Part model, mm, in its own coordinate system. A direction names the side the tool comes from. Give positions to 0.01 mm unless a question says otherwise; leave off trailing zeros. Write each loop counter-clockwise with the first axis right and the second up, starting at its lowest first coordinate (ties: lowest second). Pieces come first, ordered by that corner, then holes. Notation, with made-up numbers: M 72,81.25 L 91,81.25 A20 cw 91,117.25 Z; hole C 26,3.25 d8. An arc over 180 degrees is marked long. Answer as CSV lines item,"result". Start each with the question number.
Item 1: Wall check: L1, parallel to X at y = -10.25, z = 8.5; L2, parallel to Y at x = 2.25, z = 7.75; L3, parallel to X at y = 5.75, z = 7. Give the ranges that are in metal, low to high. Write a range as from..to.
Item 2: Pin check, flat tips, straight feed: pin 1 (4.5 mm diameter, centred on x = 10, y = -6.5, fed in from +Z); pin 2 (2 mm diameter, centred on y = 11.5, z = 7, fed in from -X); pin 3 (2 mm diameter, centred on x = -14.5, z = 6.5, fed in from +Y). Stop position of each tip, or through.
Item 3: 3-axis set-ups, long thin cutter, end or side, ignore diameter. For faces 1 (the flat face through (-13, -1, 6)), 2 (the flat face through (8.4, -5, 7.016)), 3 (the flat face through (-14, 10, 6)): which of +Z, -Z, +X, -X, +Y, -Y reach the whole face in a straight line?
Item 4: Band-saw the part on B-B, the plane x = 7. List the corners of the cut face in (y, z).
Item 5: Band-saw the part on D-D, the plane x = -3. List the corners of the cut face in (y, z).
Item 6: Two-plate mould, pull along Z, no slides. Class faces 4 (the flat face through (0, 12, 6)), 5 (the flat face through (-3, 6, 10)), 6 (the cylindrical face through (4.55, -5.08, 2.75)): +Z half, -Z half, draft (parallel to the pull), parting line (faces both ways), or undercut.
Item 7: Band-saw the part on C-C, the plane y = 6. List the corners of the cut face in (x, z), then the cut area to 3 significant figures.
Item 8: Band-saw the part on A-A, the plane y = -5. List the corners of the cut face in (x, z), then the cut area to 3 significant figures.
from build123d import *

# Parameters (mm, degrees)
F0_W      = 30
F0_H      = 26
F1_DEPTH  = 2
F3_DEPTH  = 8
F4_R      = 2.5
F5_DEPTH  = 8
F7_DEPTH  = 12
F9_DEPTH  = 5
F10_R     = 1
F11_DEPTH = 30.001


with BuildPart() as f1:
    # F0 (on Top) → F1 (new body)
    with BuildSketch(Plane.XY):
        Rectangle(F0_W, F0_H)
    extrude(amount=F1_DEPTH)

    # F2 (on face) → F3 (join)
    with BuildSketch(Plane.XY.offset(2)):
        Polygon((-15, 10), (-15, -13), (15, -13), (15, 13), (0, 13), (0, 11), (13, 11), (13, -11), (-13, -11), (-13, 10), align=None)
    extrude(amount=F3_DEPTH)

    # F4 (on face) → F5 (join, through all)
    with BuildSketch(Plane.XY.offset(2)):
        with Locations((-3, 6)):
            Circle(F4_R)
    extrude(amount=F5_DEPTH)

    # F6 (on face) → F7 (join)
    with BuildSketch(Plane(origin=(13, 0, 0), x_dir=(0, -1, 0), z_dir=(-1, 0, 0))):
        with BuildLine():
            Line((8.5, 0), (8.5, 5))
            ThreePointArc((8.5, 5), (8.3365275924, 6.0571582782), (7.8613807856, 7.0155644371))
            Line((7.8613807856, 7.0155644371), (6, 7.0155644371))
            ThreePointArc((6, 7.0155644371), (5, 2.75), (4, 7.0155644371))
            Line((4, 7.0155644371), (2.1386192144, 7.0155644371))
            ThreePointArc((2.1386192144, 7.0155644371), (1.6634724076, 6.0571582782), (1.5, 5))
            Line((1.5, 5), (1.5, 0))
            Line((1.5, 0), (8.5, 0))
        make_face()
    extrude(amount=F7_DEPTH)

    # F8 (on face) → F9 (join)
    with BuildSketch(Plane(origin=(13, 0, 0), x_dir=(0, -1, 0), z_dir=(-1, 0, 0))):
        with BuildLine():
            Line((1.5, 2), (8.5, 2))
            Line((8.5, 2), (8.5, 5))
            ThreePointArc((8.5, 5), (8.3365275924, 6.0571582782), (7.8613807856, 7.0155644371))
            Line((7.8613807856, 7.0155644371), (2.1386192144, 7.0155644371))
            ThreePointArc((2.1386192144, 7.0155644371), (1.6634724076, 6.0571582782), (1.5, 5))
            Line((1.5, 5), (1.5, 2))
        make_face()
    extrude(amount=F9_DEPTH)

    # F10 (on face) → F11 (cut, through all)
    with BuildSketch(Plane.YZ.offset(15)):
        with Locations((-5, 5)):
            Circle(F10_R)
    extrude(amount=-F11_DEPTH, mode=Mode.SUBTRACT)


solid = f1.part
Output:
1,L1,"-15..-13, 13..15"
1,L2,"-13..-11, 11..13"
1,L3,"-15..-13, -5.49..-0.51, 13..15"
2,pin 1,"z = 7.02"
2,pin 2,"x = 0"
2,pin 3,"y = 10"
3,face 1,"+Z, +Y"
3,face 2,"+Z"
3,face 3,"+Z, -X, +Y"
4,outline,"M -13,0 L 13,0 L 13,10 L 11,10 L 11,2 L -1.5,2 L -1.5,5 A3.5 ccw -2.14,7.02 L -4,7.02 A2.25 cw long -6,7.02 L -7.86,7.02 A3.5 ccw -8.5,5 L -8.5,2 L -11,2 L -11,10 L -13,10 Z"
5,outline,"M -13,0 L 13,0 L 13,2 L 8.5,2 L 8.5,10 L 3.5,10 L 3.5,2 L -11,2 L -11,10 L -13,10 Z"
6,face 4,"draft"
6,face 5,"+Z half"
6,face 6,"undercut"
7,outline,"M -15,0 L 15,0 L 15,10 L 13,10 L 13,2 L -0.5,2 L -0.5,10 L -5.5,10 L -5.5,2 L -13,2 L -13,10 L -15,10 Z"
7,area,"132 mm²"
8,outline,"M -15,0 L 15,0 L 15,4 L 8,4 L 8,2.75 L 1,2.75 L 1,2 L -13,2 L -13,4 L -15,4 Z; M -15,6 L -13,6 L -13,10 L -15,10 Z; M 8,6 L 15,6 L 15,10 L 13,10 L 13,7.02 L 8,7.02 Z"
8,area,"104 mm²"
